The model under review builds one solid part; all positions refer to its coordinate system, in mm. A direction names the side the tool comes from. Coordinates: 2 decimals unless noted, no trailing zeros. Write each loop counter-clockwise with the first axis right and the second up, starting at its lowest first coordinate (ties: lowest second). Pieces come first, ordered by that corner, then holes. Notation, with made-up numbers: (31, 29.25) - (39, 29.25) arc R19 cw to (39, 42.25) - close; hole circle Ø7 at (-22, -1.5). An arc over 180 degrees is marked (long way). Put each result on its own line as item: value. Start each with the question number.
Item 1: Consider section C-C on x = 1. Give the boundary of the cut face in (y, z).
Item 2: To check wall thickness, follow L1, parallel to Y at x = 0, z = 6.7; L2, parallel to X at y = -2.75, z = 4.25 (3 decimals); L3, parallel to Y at x = 0, z = 5.15. State the ranges of each line that lie inside material, in increasing order. Write a range as [from, to].
Item 3: For pin 1 (1.5 mm diameter, centred on x = 0, y = -1.5, fed in from +Z); pin 2 (1 mm diameter, centred on x = -3, y = 2, fed in from -Z); pin 3 (1.8 mm diameter, centred on x = 1, y = 0.5, fed in from -Z), all flat-tipped, find the tip position at first contact; note any pin that passes through.
Item 4: Consider section B-B on z = 2.75. Give the boundary of the cut face in (x, y).
Item 5: Consider section A-A on y = 0. Give the boundary of the cut face in (x, z).
Item 6: Machinability: for faces 4 (the face through (-0.54, -2.44, 6.92)), 5 (the face through (0.01, 1.12, 2.46)), 6 (the face through (2, -2, 8.5)), which of the approach directions +Z, -Z, +X, -X, +Y, -Y give a long, thin tool a straight path to every point of the face, cutting with its end or side? Answer none if there is none.
Item 7: Mouldability with a two-part tool opening along X and no side actions: class faces 1 (the face through (0, -2, 0)), 2 (the face through (-0.01, -1.12, 2.46)), 3 (the face through (-1.08, -4.88, 4.19)) as pulls with the +X half, pulls with the -X half, needs draft (parallel to the pull), parting line crosses it, or undercut.
Item 8: Consider section D-D on y = 2. Give the boundary of the cut face in (x, z).
```python
from build123d import *

# Parameters (mm, degrees)
SKETCH2_R           = 5
BOSS_EXTRUDE1_DEPTH = 8.5
CUT_EXTRUDE1_DEPTH  = 5
SKETCH3_R           = 2.5
CUT_EXTRUDE2_DEPTH  = 3.2
SKETCH5_R           = 0.35
CUT_EXTRUDE4_DEPTH  = 1


with BuildPart() as part:
    # Sketch2 → Boss-Extrude1 (new body)
    with BuildSketch(Plane.XY):
        Circle(SKETCH2_R)
    extrude(amount=BOSS_EXTRUDE1_DEPTH)

    # Sketch1 → Cut-Extrude1 (cut)
    with BuildSketch(Plane.XY):
        with BuildLine():
            Line((-0.447213595, 1.394427191), (-1.135934639, 2.771869278))
            ThreePointArc((-1.135934639, 2.771869278), (-1.447076632, 3.029390861), (-1.847006274, 2.972972894))
            ThreePointArc((-1.847006274, 2.972972894), (-3.5, 0), (-1.847006274, -2.972972894))
            ThreePointArc((-1.847006274, -2.972972894), (-1.447076632, -3.029390861), (-1.135934639, -2.771869278))
            Line((-1.135934639, -2.771869278), (-0.447213595, -1.394427191))
            ThreePointArc((-0.447213595, -1.394427191), (0, -1.118033989), (0.447213595, -1.394427191))
            Line((0.447213595, -1.394427191), (1.135934639, -2.771869278))
            ThreePointArc((1.135934639, -2.771869278), (1.447076632, -3.029390861), (1.847006274, -2.972972894))
            ThreePointArc((1.847006274, -2.972972894), (3.5, 0), (1.847006274, 2.972972894))
            ThreePointArc((1.847006274, 2.972972894), (1.447076632, 3.029390861), (1.135934639, 2.771869278))
            Line((1.135934639, 2.771869278), (0.447213595, 1.394427191))
            ThreePointArc((0.447213595, 1.394427191), (0, 1.118033989), (-0.447213595, 1.394427191))
        make_face()
    extrude(amount=CUT_EXTRUDE1_DEPTH, mode=Mode.SUBTRACT)

    # Sketch3 → Cut-Extrude2 (cut)
    with BuildSketch(Plane.XY.offset(8.5)):
        Circle(SKETCH3_R)
    extrude(amount=-CUT_EXTRUDE2_DEPTH, mode=Mode.SUBTRACT)

    # Sketch5 → Cut-Extrude4 (cut)
    with BuildSketch(Plane(origin=(0, 0, 5), x_dir=(-1, 0, 0), z_dir=(0, 0, -1))):
        Circle(SKETCH5_R)
    extrude(amount=-CUT_EXTRUDE4_DEPTH, mode=Mode.SUBTRACT)


solid = part.part
```
Report:
1. outline: (-4.9, 0) - (-2.5, 0) - (-2.5, 5) - (2.5, 5) - (2.5, 0) - (4.9, 0) - (4.9, 8.5) - (2.29, 8.5) - (2.29, 5.3) - (-2.29, 5.3) - (-2.29, 8.5) - (-4.9, 8.5) - close
2. L1: [-5, -2.5], [2.5, 5]
2. L2: [-4.176, -2.165], [-1.125, 1.125], [2.165, 4.176]
2. L3: [-5, -0.35], [0.35, 5]
3. pin 1: z = 5.3
3. pin 2: z = 0
3. pin 3: z = 5
4. outline: circle Ø10 at (0, 0); hole (-1.85, -2.97) arc R0.5 ccw to (-1.14, -2.77) - (-0.45, -1.39) arc R0.5 cw to (0.45, -1.39) - (1.14, -2.77) arc R0.5 ccw to (1.85, -2.97) arc R3.5 ccw to (1.85, 2.97) arc R0.5 ccw to (1.14, 2.77) - (0.45, 1.39) arc R0.5 cw to (-0.45, 1.39) - (-1.14, 2.77) arc R0.5 ccw to (-1.85, 2.97) arc R3.5 ccw to start
5. outline: (-5, 0) - (-3.5, 0) - (-3.5, 5) - (-0.35, 5) - (-0.35, 5.3) - (-2.5, 5.3) - (-2.5, 8.5) - (-5, 8.5) - close; (0.35, 5) - (3.5, 5) - (3.5, 0) - (5, 0) - (5, 8.5) - (2.5, 8.5) - (2.5, 5.3) - (0.35, 5.3) - close
6. face 4: +Z
6. face 5: -Z
6. face 6: +Z, +X, -X, +Y, -Y
7. face 1: needs draft
7. face 2: undercut
7. face 3: parting line crosses it
8. outline: (-4.58, 0) - (-2.87, 0) - (-2.87, 5) - (-0.75, 5) - (-0.75, 0) - (0.75, 0) - (0.75, 5) - (2.87, 5) - (2.87, 0) - (4.58, 0) - (4.58, 8.5) - (1.5, 8.5) - (1.5, 5.3) - (-1.5, 5.3) - (-1.5, 8.5) - (-4.58, 8.5) - close
